```python
from build123d import *

# Parameters (mm, degrees)
F0_W     = 1.65
F0_H     = 0.9
F1_DEPTH = 2
F2_DEPTH = 9
F3_R     = 1


with BuildPart() as f1:
    # F0 (on Top) → F1 (new body)
    with BuildSketch(Plane.XY):
        Polygon((9.25, -2.175), (9.25, 4.675), (-9.25, 4.675), (-9.25, -2.175), (-9.25, -5.575), (3.95, -5.575), (5.6, -5.575), (9.25, -5.575), align=None)
        Polygon((-8.75, -2.175), (-8.75, 4.175), (8.75, 4.175), (8.75, -2.175), (8.75, -5.075), (5.6, -5.075), (3.95, -5.075), (-8.75, -5.075), align=None, mode=Mode.SUBTRACT)
        Polygon((8.75, 4.175), (-8.75, 4.175), (-8.75, -2.175), (-8.75, -5.075), (3.95, -5.075), (5.6, -5.075), (8.75, -5.075), (8.75, -2.175), align=None)
        Polygon((-6.75, 2.175), (6.75, 2.175), (6.75, -2.175), (5.6, -2.175), (5.6, -3.075), (3.95, -3.075), (3.95, -2.175), (-3.95, -2.175), (-3.95, -3.075), (-5.6, -3.075), (-5.6, -2.175), (-6.75, -2.175), align=None, mode=Mode.SUBTRACT)
        Polygon((6.75, -2.175), (6.75, 2.175), (-6.75, 2.175), (-6.75, -2.175), (-5.6, -2.175), (-3.95, -2.175), (3.95, -2.175), (5.6, -2.175), align=None)
        with Locations((-4.775, -2.625)):
            Rectangle(F0_W, F0_H)
        with Locations((4.775, -2.625)):
            Rectangle(F0_W, F0_H)
    extrude(amount=F1_DEPTH)

    # F0 (on Top) → F2 (join)
    with BuildSketch(Plane.XY):
        Polygon((8.75, 4.175), (-8.75, 4.175), (-8.75, -2.175), (-8.75, -5.075), (3.95, -5.075), (5.6, -5.075), (8.75, -5.075), (8.75, -2.175), align=None)
        Polygon((-6.75, 2.175), (6.75, 2.175), (6.75, -2.175), (5.6, -2.175), (5.6, -3.075), (3.95, -3.075), (3.95, -2.175), (-3.95, -2.175), (-3.95, -3.075), (-5.6, -3.075), (-5.6, -2.175), (-6.75, -2.175), align=None, mode=Mode.SUBTRACT)
    extrude(amount=F2_DEPTH)

    # F3
    f3_edges = [f1.edges().sort_by_distance(p)[0] for p in [
        (-9.25, -5.575, 1),
        (-8.75, -5.075, 5.5),
        (-9.25, 4.675, 1),
        (-8.75, 4.175, 5.5),
        (8.75, -5.075, 5.5),
        (9.25, -5.575, 1),
        (8.75, 4.175, 5.5),
        (9.25, 4.675, 1),
        (0, -5.075, 9),
        (-8.75, -0.45, 9),
        (0, 4.175, 9),
        (8.75, -0.45, 9),
    ]]
    fillet(f3_edges, radius=F3_R)


solid = f1.part
```
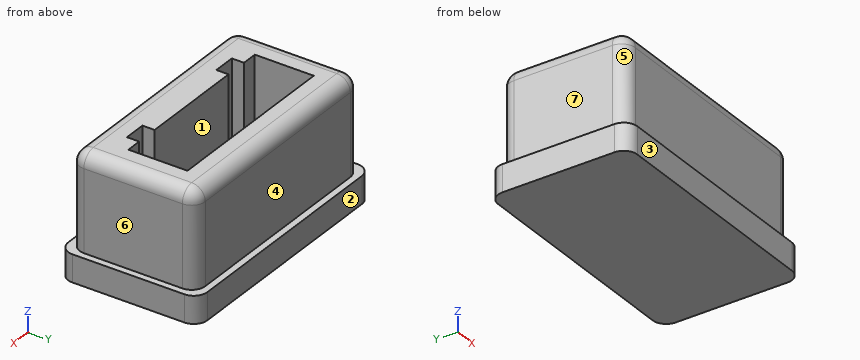
Geometry check sheet. Reference: the model listing, model coordinates, mm. Face numbers are marked on the shaded views. A direction names the side the tool comes from. Give positions to 0.01 mm unless a question says otherwise; leave off trailing zeros. Order: outer loops, then holes, each group sorted by start corner. A loop starts at its lowest first (then second) coordinate and runs counter-clockwise, first axis right, second up. Notation, with made-up numbers: (-0.5, -7.75) - (17.5, -7.75) arc R31 ccw to (17.5, 19.25) - close; hole circle Ø1 at (58, 42.5). An arc over 180 degrees is marked (long way). Write item = value, one per line. Start each with the question number.
1) Section check B-B (x = 1.5). Enter the section's corners in (y, z) (3 decimals).
2) Gauge pin test, flat ends, axial feed: pin 1 Ø3 at (x, z) = (2.5, 4) entering from -Y (3 decimals); pin 2 Ø4 at (y, z) = (3, 3) entering from -X; pin 3 Ø1.8 at (x, z) = (-5, 7) entering from +Y (3 decimals); pin 4 Ø2 at (y, z) = (-0.5, 5.5) entering from -X. Record the tip position at first contact, or that the pin passes through.
3) Section check A-A (z = 6). Enter the section's corners in (x, y) (3 decimals), then the cut area to 3 significant figures.
4) Scan lines: L1, parallel to X at y = -3, z = 6.25; L2, parallel to Y at x = -2, z = 3 (3 decimals); L3, parallel to X at y = -2, z = 7.75. Record each from-to range of solid material in increasing order.
5) Section check D-D (y = 2.75). Enter the section's corners in (x, z), then the cut area to 3 significant figures.
6) Draft check along Y on the marked faces 1, 2 and 3. Enter one of: released by +Y, released by -Y, zero draft, split by the parting line, or undercut.
7) Access from +Z, -Z, +X, -X, +Y, -Y to the whole of each face (thin tool, end or side, straight path). Record for the marked faces 4, 5, 6 and 7.
8) Section check C-C (y = -1.25). Enter the section's corners in (x, z), then the cut area to 3 significant figures.
Geometry check:
q1.outline = (-5.575, 0) - (4.675, 0) - (4.675, 2) - (4.175, 2) - (4.175, 8) arc R1 ccw to (3.175, 9) - (2.175, 9) - (2.175, 2) - (-2.175, 2) - (-2.175, 9) - (-4.075, 9) arc R1 ccw to (-5.075, 8) - (-5.075, 2) - (-5.575, 2) - close
q2.pin_1 = -5.075
q2.pin_2 = -9.25
q2.pin_3 = 4.175
q2.pin_4 = -8.75
q3.outline = (-8.75, -4.075) arc R1 ccw to (-7.75, -5.075) - (7.75, -5.075) arc R1 ccw to (8.75, -4.075) - (8.75, 3.175) arc R1 ccw to (7.75, 4.175) - (-7.75, 4.175) arc R1 ccw to (-8.75, 3.175) - close; hole (-6.75, -2.175) - (-5.6, -2.175) - (-5.6, -3.075) - (-3.95, -3.075) - (-3.95, -2.175) - (3.95, -2.175) - (3.95, -3.075) - (5.6, -3.075) - (5.6, -2.175) - (6.75, -2.175) - (6.75, 2.175) - (-6.75, 2.175) - close
q3.area = 99.3 mm2
q4.L1 = -8.75 to -5.6, -3.95 to 3.95, 5.6 to 8.75
q4.L2 = -5.075 to -2.175, 2.175 to 4.175
q4.L3 = -8.75 to -6.75, 6.75 to 8.75
q5.outline = (-9.25, 0) - (9.25, 0) - (9.25, 2) - (8.75, 2) - (8.75, 8) arc R1 ccw to (7.75, 9) - (-7.75, 9) arc R1 ccw to (-8.75, 8) - (-8.75, 2) - (-9.25, 2) - close
q5.area = 159 mm2
q6.face_1 = undercut
q6.face_2 = released by +Y
q6.face_3 = released by -Y
q7.face_4 = +Z, +X, -X, +Y
q7.face_5 = +Z, -X, -Y
q7.face_6 = +Z, +X, +Y, -Y
q7.face_7 = +Z, -X, +Y, -Y
q8.outline = (-9.25, 0) - (9.25, 0) - (9.25, 2) - (8.75, 2) - (8.75, 8) arc R1 ccw to (7.75, 9) - (6.75, 9) - (6.75, 2) - (-6.75, 2) - (-6.75, 9) - (-7.75, 9) arc R1 ccw to (-8.75, 8) - (-8.75, 2) - (-9.25, 2) - close
q8.area = 64.6 mm2
